Geometry check sheet. Reference: drawing and pictorial views, mm from the part's lowest x, y, z. A direction names the side the tool comes from. Round coordinates to 2 decimals unless told otherwise and drop trailing zeros. Write each loop counter-clockwise with the first axis right and the second up, starting at its lowest first coordinate (ties: lowest second). Pieces come first, ordered by that corner, then holes. Notation, with made-up numbers: M 4,41.25 L 9,41.25 A26 ccw 9,74.25 Z; hole C 43.5,54 d9. An arc over 180 degrees is marked long. Answer in a Markdown table with one row per item. Add a question column.
1. Draft check along X on the marked faces 1, 2, 3 and 4. Enter one of: pulls with the +X half, pulls with the -X half, needs draft (parallel to the pull), parting line crosses it, or undercut.
2. Sectioned sample at B-B on z = 14. Record the cut outline in (x, y), plus the area to 3 significant figures.
3. Sectioned sample at A-A on y = 2. Record the cut outline in (x, z).
4. Go/stop test with flat-tipped pins: pin 1 Ø14 at (y, z) = (13, 21) entering from -X; pin 2 Ø6 at (y, z) = (3, 21) entering from +X; pin 3 Ø3 at (x, y) = (50, 16) entering from +Z. Record where each tip stops, or that it passes through.
5. Material ranges on probe 1 along X at (y, z) = (18, 18.25); probe 2 along Y at (x, z) = (56, 8) (1 decimal); probe 3 along Y at (x, z) = (8, 11.75) (1 decimal), recorded low to high.
6. Sectioned sample at C-C on x = 45.5. Record the cut outline in (y, z), plus the area to 3 significant figures.
7. Set-up check for the marked faces 5, 6 and 7: record each of +Z, -Z, +X, -X, +Y, -Y from which the full face is reachable in a straight line by a thin tool's end or side.
8. Sectioned sample at D-D on z = 5.5. Record the cut outline in (x, y), plus the area to 3 significant figures.
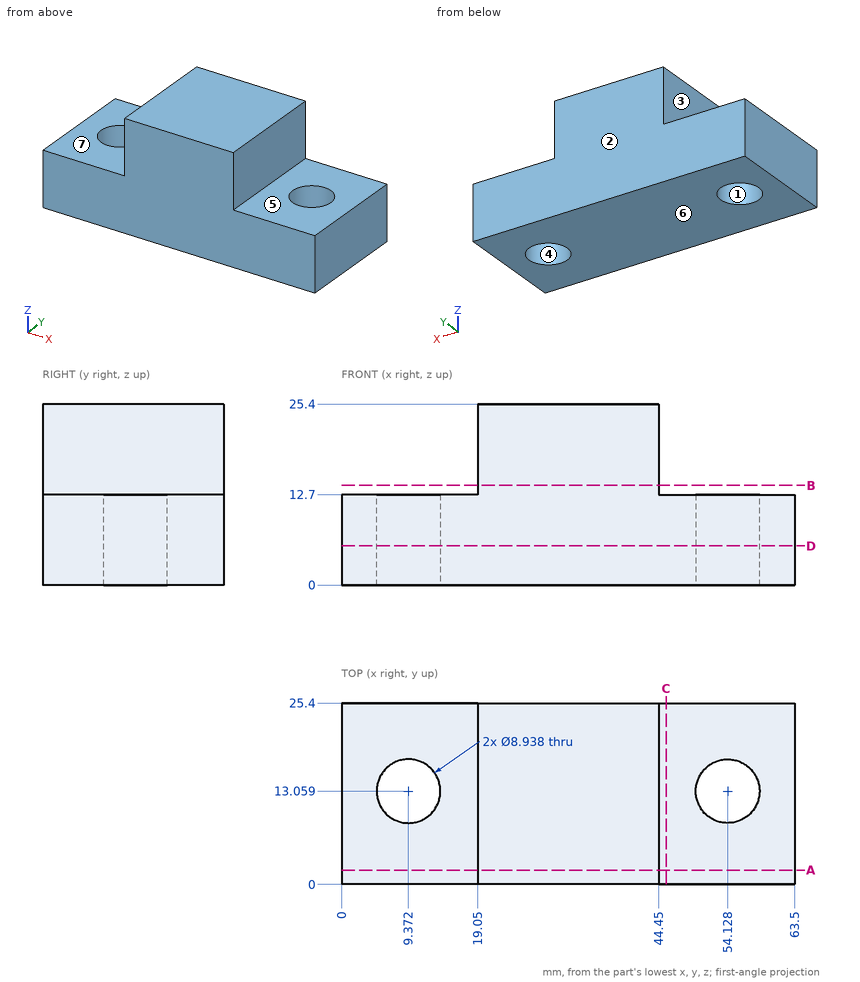
Geometry check:
| question | item | result |
|---|---|---|
| 1 | face 1 | undercut |
| 1 | face 2 | needs draft |
| 1 | face 3 | pulls with the -X half |
| 1 | face 4 | undercut |
| 2 | outline | M 19.05,0 L 44.45,0 L 44.45,25.4 L 19.05,25.4 Z |
| 2 | area | 645 mm2 |
| 3 | outline | M 0,0 L 63.5,0 L 63.5,12.7 L 44.45,12.7 L 44.45,25.4 L 19.05,25.4 L 19.05,12.7 L 0,12.7 Z |
| 4 | pin 1 | stops at x = 19.05 |
| 4 | pin 2 | stops at x = 44.45 |
| 4 | pin 3 | stops at z = 12.7 |
| 5 | probe 1 | x = 19.05 to 44.45 |
| 5 | probe 2 | y = 0 to 9, 17.1 to 25.4 |
| 5 | probe 3 | y = 0 to 8.8, 17.3 to 25.4 |
| 6 | outline | M 0,0 L 25.4,0 L 25.4,12.7 L 0,12.7 Z |
| 6 | area | 323 mm2 |
| 7 | face 5 | +Z, +X, +Y, -Y |
| 7 | face 6 | -Z, +X, -X, +Y, -Y |
| 7 | face 7 | +Z, -X, +Y, -Y |
| 8 | outline | M 0,0 L 63.5,0 L 63.5,25.4 L 0,25.4 Z; hole C 9.37,13.06 d8.94; hole C 54.13,13.06 d8.94 |
| 8 | area | 1,490 mm2 |
